Autodesk Fusion 360 part; units mm, degrees
sketch "Sketch1" plane through (0, 0, 0) normal (0, 1, 0) x (1, 0, 0)
  line L0 (-25, 30) -> (45, 30)
  line L1 (45, 30) -> (45, -40)
  line L2 (45, -40) -> (-25, -40)
  line L3 (-25, -40) -> (-25, 30)
  dimension "d1" = 70
  dimension "d2" = 70
extrude "Extrude1" add sketch "Sketch1" against normal blind 3
sketch "Sketch2" plane through (0, 0, 0) normal (0, 1, 0) x (-1, 0, 0)
  line L0 (25, 40) -> (-45, 40)
  line L1 (-45, 40) -> (-45, -30)
  line L2 (-45, -30) -> (25, -30)
  line L3 (25, -30) -> (25, 40)
  line L4 (25, 35) -> (-45, 35)
  line L5 (-45, 35) -> (-45, 40)
  line L6 (-45, 40) -> (25, 40)
  line L7 (25, 40) -> (25, 35)
sketch "Sketch3" plane through (0, 0, 0) normal (0, 1, 0) x (-1, 0, 0)
  line L0 (25, -30) -> (-45, -30)
  line L1 (-45, -30) -> (-45, -25)
  line L2 (-45, -25) -> (25, -25)
  line L3 (25, -25) -> (25, -30)
extrude "Extrude2" add sketch "Sketch2" sketch "Sketch3" along normal blind 50 contours L0 L1 L3 L4 L5 L6 L7 of sketch 2
sketch "Sketch4" plane through (0, 0, -25) normal (0, 0, 1) x (1, 0, 0)
  line L0 (-25, 0) -> (45, 0)
  line L1 (45, 0) -> (45, 50)
  line L2 (45, 50) -> (-25, 50)
  line L3 (-25, 50) -> (-25, 0)
  line L4 (-25, 50) -> (45, 50)
  line L5 (45, 50) -> (45, 47)
  line L6 (45, 47) -> (-25, 47)
  line L7 (-25, 47) -> (-25, 50)
extrude "Extrude3" add sketch "Sketch4" along normal blind 60 contours L1 L2 L3 L4 L5 L6 L7
sketch "Sketch5" plane through (0, 50, 0) normal (0, 1, 0) x (-1, 0, 0)
  line L0 (-45, 40) -> (-45, -30)
  line L1 (-45, -30) -> (25, -30)
  line L2 (25, -30) -> (25, 40)
  line L3 (25, 40) -> (-45, 40)
  line L4 (25, 40) -> (22, 40)
  line L5 (22, 40) -> (22, -30)
  line L6 (22, -30) -> (25, -30)
  line L7 (25, -30) -> (25, 40)
  dimension "d9" = 3
sketch "Sketch6" plane through (0, 50, 0) normal (0, 1, 0) x (-1, 0, 0)
  line L0 (-45, 40) -> (-42, 40)
  line L1 (-42, 40) -> (-42, -30)
  line L2 (-42, -30) -> (-45, -30)
  line L3 (-45, -30) -> (-45, 40)
  dimension "d10" = 3
extrude "Extrude4" add sketch "Sketch6" sketch "Sketch5" along normal blind 50 of sketch 2 contours L1 L2 L3 L4 L5 L6 L7
sketch "Sketch7" plane through (-22, 0, 0) normal (1, 0, 0) x (0, 0, -1)
  line L0 (-40, 50) -> (30, 50)
  line L1 (30, 50) -> (30, 100)
  line L2 (30, 100) -> (-40, 100)
  line L3 (-40, 100) -> (-40, 50)
  line L4 (-40, 100) -> (30, 100)
  line L5 (30, 100) -> (30, 97)
  line L6 (30, 97) -> (-40, 97)
  line L7 (-40, 97) -> (-40, 100)
  dimension "d13" = 3
extrude "Extrude5" add sketch "Sketch7" along normal blind 64 contours L1 L2 L3 L4 L5 L6 L7
sketch "Sketch8" plane through (-25, 0, 0) normal (-1, 0, 0) x (0, 0, 1)
  line L0 (-30, 100) -> (-30, -3)
  line L1 (-30, -3) -> (40, -3)
  line L2 (40, -3) -> (40, 100)
  line L3 (40, 100) -> (-30, 100)
  line L4 (-25, 47) -> (35, 47)
  line L5 (35, 47) -> (35, 0)
  line L6 (35, 0) -> (-25, 0)
  line L7 (-25, 0) -> (-25, 47)
  line L8 (-25, 50) -> (35, 50)
  line L9 (35, 50) -> (35, 97)
  line L10 (35, 97) -> (-25, 97)
  line L11 (-25, 97) -> (-25, 50)
  dimension "d16" = 60
  dimension "d17" = 47
extrude "Extrude6" cut sketch "Sketch8" against normal blind 80 contours L8 L9 L10 L11
Design review of the part built by this model. Coordinates are the model's own, in mm. A direction names the side the tool comes from. Give positions to 0.01 mm unless a question says otherwise; leave off trailing zeros. Order: outer loops, then holes, each group sorted by start corner. A loop starts at its lowest first (then second) coordinate and runs counter-clockwise, first axis right, second up. Notation, with made-up numbers: (-15.75, 0) - (25.25, 0) arc R20 cw to (25.25, 13) - close; hole circle Ø6 at (-10.75, 19.5). An arc over 180 degrees is marked (long way). Use CSV: the item, a comma, the result in double quotes. Start each with the question number.
Q1. Machinability: for faces 4 (the face through (43, 73, 35)), 5 (the face through (42, 73, -27)), 6 (the face through (10, -3, 5)), which of the approach directions +Z, -Z, +X, -X, +Y, -Y give a long, thin tool a straight path to every point of the face, cutting with its end or side? Answer none if there is none.
Q2. Draft analysis for pull direction X (two halves, no side actions). For faces 1 (the face through (10, 50, 5)), 2 (the face through (10, 23, 35)), 3 (the face through (-25, 49, 5)), state which applies: pulls with the +X half, pulls with the -X half, needs draft (parallel to the pull), parting line crosses it, or undercut.
Q3. Take a section at A-A (y = 66.5). State the section outline as (x, z) points.
Q4. For P1, Ø12, axis at x = 30.5, y = 76, coming from the -Z side, flat-tipped, find the tip position at first contact; note if it passes through.
Q5. Take a section at C-C (x = -18.5). State the section outline as (y, z) points, and give its area (3 significant figures).
Q6. Take a section at D-D (y = 18). State the section outline as (x, z) points.
Q7. Take a section at B-B (z = -19.5). State the section outline as (x, y) points.
Q8. For line 1 (Y direction, x = 23.5, z = -2); line 2 (Z direction, x = -7.5, y = 10.5); line 3 (Y direction, x = 19.5, z = -26), list the stretches that pass through material, from the lowest coordinate up.
Calculated:
1,face 4,"+X, -X"
1,face 5,"+Z, -Z"
1,face 6,"+Z, -Z, +X, -X, -Y"
2,face 1,"undercut"
2,face 2,"needs draft"
2,face 3,"pulls with the -X half"
3,outline,"(-25, -30) - (-22, -30) - (-22, -25) - (-25, -25) - close; (-25, 35) - (-22, 35) - (-22, 40) - (-25, 40) - close; (42, -30) - (45, -30) - (45, -25) - (42, -25) - close; (42, 35) - (45, 35) - (45, 40) - (42, 40) - close"
4,P1,"passes through"
5,outline,"(-3, -30) - (50, -30) - (50, 40) - (-3, 40) - close; (97, -30) - (100, -30) - (100, 40) - (97, 40) - close; hole (0, -25) - (47, -25) - (47, 35) - (0, 35) - close"
5,area,"1,100 mm²"
6,outline,"(-25, -30) - (45, -30) - (45, -25) - (-25, -25) - close; (-25, 35) - (45, 35) - (45, 40) - (-25, 40) - close"
7,outline,"(-25, -3) - (45, -3) - (45, 0) - (-25, 0) - close; (-25, 47) - (45, 47) - (45, 50) - (-25, 50) - close; (-25, 97) - (45, 97) - (45, 100) - (-25, 100) - close"
8,line 1,"y = -3 to 0, 47 to 50, 97 to 100"
8,line 2,"z = -30 to -25, 35 to 40"
8,line 3,"y = -3 to 50, 97 to 100"
